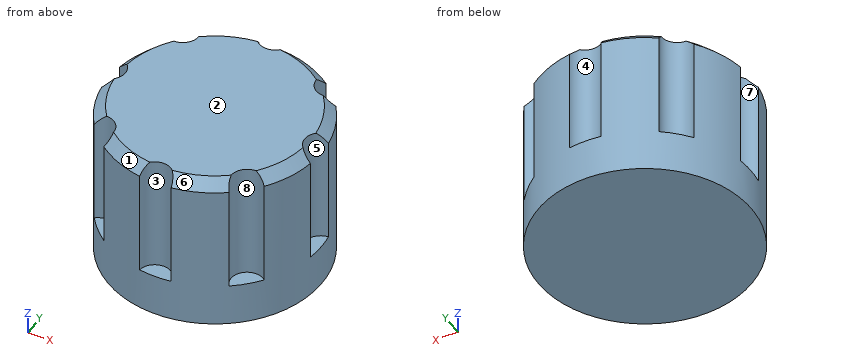
```python
from build123d import *

# Parameters (mm, degrees)
CYLINDER001_R     = 1.5
CYLINDER001_DEPTH = 20
ARRAY_COUNT       = 8
CYLINDER_R        = 10
CYLINDER_DEPTH    = 15
CHAMFER_SIZE      = 1


with BuildPart() as array:
    # Cylinder001 → Cylinder001 (new body)
    with BuildSketch(Plane.XY.offset(4)):
        Circle(CYLINDER001_R)
    extrude(amount=CYLINDER001_DEPTH)

    # Array: Array ×8 about axis
    array_axis = Axis((10, 0, 0), (0, 0, 1))


with BuildPart() as array_1:
    add(array.part)
    for i in range(1, ARRAY_COUNT):
        add(array.part.rotate(array_axis, i * 360 / ARRAY_COUNT))


with BuildPart() as array_2:
    # Array placement: moved
    add(array_1.part.moved(Location((-10, 0, 0))))


with BuildPart() as chamfer_body:
    # Cylinder → Cylinder (new body)
    with BuildSketch(Plane.XY):
        Circle(CYLINDER_R)
    extrude(amount=CYLINDER_DEPTH)

    # Cut: cut Array
    add(array_2.part, mode=Mode.SUBTRACT)

    # Chamfer
    chamfer_edges = [chamfer_body.edges().sort_by_distance(p)[0] for p in [
        (9.238795, -3.826834, 15),
        (3.826834, -9.238795, 15),
        (-3.826834, -9.238795, 15),
        (-9.238795, -3.826834, 15),
        (-9.238795, 3.826834, 15),
        (-3.826834, 9.238795, 15),
        (3.826834, 9.238795, 15),
        (9.238795, 3.826834, 15),
    ]]
    chamfer(chamfer_edges, length=CHAMFER_SIZE)


solid = chamfer_body.part
```
Input: part model. Units: mm. Frame: model coordinates. Face numbers are marked on the shaded views. A direction names the side the tool comes from. Round coordinates to 2 decimals unless told otherwise and drop trailing zeros. Write each loop counter-clockwise with the first axis right and the second up, starting at its lowest first coordinate (ties: lowest second). Pieces come first, ordered by that corner, then holes. Notation, with made-up numbers: (61.5, 56) - (75.5, 56) arc R17 ccw to (75.5, 68) - close; hole circle Ø6 at (39.5, -35). An arc over 180 degrees is marked (long way). Write item = value, one per line.
(1) Access query for the marked faces 5, 6, 7 and 8. Directions: +Z, -Z, +X, -X, +Y, -Y. A direction counts if a zero-diameter tool reaches every point of the face in a straight line with its end or side. Return the directions, or none.
Geometry check:
face_5 = +Z, +X
face_6 = +Z, +X, -Y
face_7 = +Z, -X
face_8 = +Z
(2) Pull-direction query (X, two-part tool) for the marked faces 1, 2, 3 and 4; classes: +X half, -X half, draft (parallel to the pull), parting line (faces both ways), or undercut.
Geometry check:
face_1 = -X half
face_2 = draft
face_3 = undercut
face_4 = undercut
(3) Contact query for flat-ended pins moving along their axis: pin 1 Ø4 at (x, z) = (7, 7.5) entering from +Y; pin 2 Ø1.2 at (x, y) = (7.5, -6.5) entering from +Z; pin 3 Ø6 at (y, z) = (4.5, 7.5) entering from -X. Output: stop coordinate, or through.
Geometry check:
pin_1 = 8.66
pin_2 = 4
pin_3 = -9.89
(4) Section query A-A on x = 0. Output: boundary loops of the cut face in (y, z), then the cut area to 3 significant figures.
Geometry check:
outline = (-10, 0) - (10, 0) - (10, 4) - (8.5, 4) - (8.5, 15) - (-8.5, 15) - (-8.5, 4) - (-10, 4) - close
area = 267 mm^2
(5) Material intervals for probe 1 along Y at (x, z) = (5.75, 6.75); probe 2 along Z at (x, y) = (7, -7); probe 3 along Y at (x, z) = (2.5, 1), sorted ascending.
Geometry check:
probe_1 = -8.18 to -7.78, -6.36 to 6.36, 7.78 to 8.18
probe_2 = 0 to 4
probe_3 = -9.68 to 9.68
(6) Section query D-D on z = 1.25. Output: boundary loops of the cut face in (x, y), then the cut area to 3 significant figures.
Geometry check:
outline = circle Ø20 at (0, 0)
area = 314 mm^2
